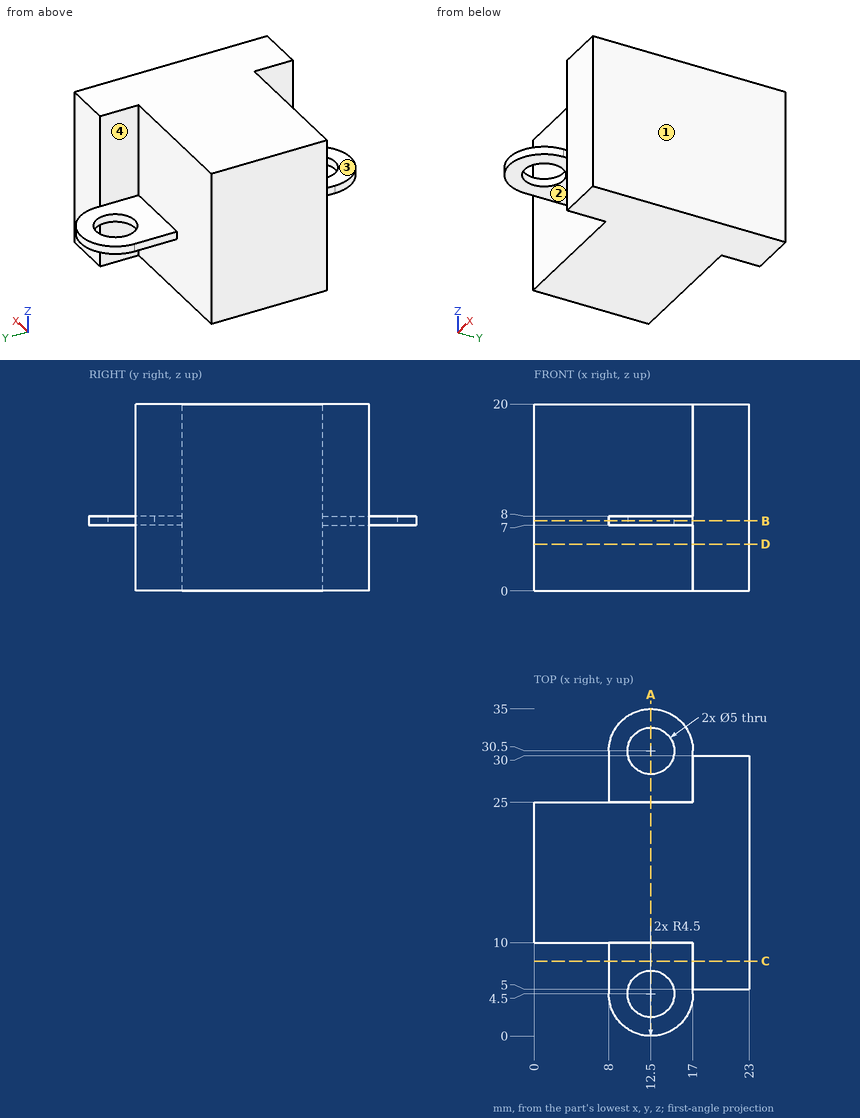
Here's the drawing with two shaded views (mm, measured from the low corner). I have some questions. A direction names the side the tool comes from. Round coordinates to 2 decimals unless told otherwise and drop trailing zeros. Loops run counter-clockwise (first coordinate to the right, second up) from the corner with the lowest first, then second, coordinate; pieces in that order, holes last.
Item 1: Will these pins go through, and if not, where does the flat tip stop? pin 1 Ø1.5 at (y, z) = (7, 2) entering from -X; pin 2 Ø8 at (x, y) = (12.5, 30.5) entering from +Z; pin 3 Ø2.5 at (x, y) = (11, 30) entering from -Z.
Item 2: Suppose I cut it at C-C, the plane y = 8. Write out the boundary of the cut face in (x, z).
Item 3: Suppose I cut it at B-B, the plane z = 7.5. Write out the boundary of the cut face in (x, y), then the cut area to 3 significant figures.
Item 4: Suppose I cut it at A-A, the plane x = 12.5. Write out the boundary of the cut face in (y, z).
Item 5: Which directions (+Z, -Z, +X, -X, +Y, -Y) give clear straight access to the entire face, cutting with the end or side of a thin tool? Please do the marked faces 1, 2, 3 and 4.
Item 6: Please list where these lines run through material, in increasing order: L1, parallel to Y at x = 12.5, z = 7.2; L2, parallel to X at y = 4.5, z = 7.6; L3, parallel to X at y = 7, z = 4.25.
Item 7: Suppose I cut it at D-D, the plane z = 5. Write out the boundary of the cut face in (x, y), then the cut area to 3 significant figures.
Reported:
1. pin 1: stops at x = 17
1. pin 2: stops at z = 8
1. pin 3: stops at z = 7
2. outline: (8, 7) - (17, 7) - (17, 0) - (23, 0) - (23, 20) - (17, 20) - (17, 8) - (8, 8) - close
3. outline: (0, 10) - (8, 10) - (8, 4.5) arc R4.5 ccw to (17, 4.5) - (17, 5) - (23, 5) - (23, 30) - (17, 30) - (17, 30.5) arc R4.5 ccw to (8, 30.5) - (8, 25) - (0, 25) - close; hole circle Ø5 at (12.5, 4.5); hole circle Ø5 at (12.5, 30.5)
3. area: 528 mm2
4. outline: (0, 7) - (2, 7) - (2, 8) - (0, 8) - close; (7, 7) - (10, 7) - (10, 0) - (25, 0) - (25, 7) - (28, 7) - (28, 8) - (25, 8) - (25, 20) - (10, 20) - (10, 8) - (7, 8) - close; (33, 7) - (35, 7) - (35, 8) - (33, 8) - close
5. face 1: +Z, -Z, +X, +Y, -Y
5. face 2: -Z, -X, -Y
5. face 3: +Z, -X, -Y
5. face 4: +Z, -X, +Y
6. L1: y = 0 to 2, 7 to 28, 33 to 35
6. L2: x = 8 to 10, 15 to 17
6. L3: x = 17 to 23
7. outline: (0, 10) - (17, 10) - (17, 5) - (23, 5) - (23, 30) - (17, 30) - (17, 25) - (0, 25) - close
7. area: 405 mm2
